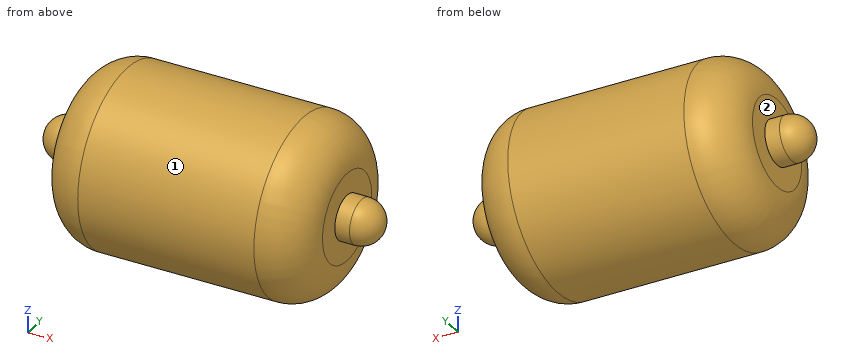
Autodesk Inventor part; units mm, degrees
ref_plane "YZ Plane" through (0, 0, 0) normal (1, 0, 0) x (0, 1, 0)
ref_plane "XZ Plane" through (0, 0, 0) normal (0, 1, 0) x (-1, 0, 0)
ref_plane "XY Plane" through (0, 0, 0) normal (0, 0, 1) x (1, 0, 0)
sketch "Sketch1" plane through (0, 0, 0) normal (0, 0, 1) x (1, 0, 0)
  line L0 (-9, -6) -> (9, -6)
  line L1 (9, -6) -> (9, 6)
  line L2 (9, 6) -> (-9, 6)
  line L3 (-9, 6) -> (-9, 0)
  line L4 (-9, -6) -> (9, 6) construction
  line L5 (9, -6) -> (-9, 6) construction
  line L6 (-9, 0) -> (9, 0)
  point P0 (0, 0)
  dimension "d0" = 18
  dimension "d1" = 12
revolve "Revolution1" add sketch "Sketch1" angle 360 about axis through (-9, 0, 0) along (1, 0, 0)
sketch "Sketch2" plane through (9, 0, 0) normal (1, 0, 0) x (0, 0, -1)
  circle A0 centre (0, 0) radius 1.5
  dimension "d3" = 3
extrude "Extrusion1" add sketch "Sketch2" along normal blind 2.5
fillet "Fillet1" radius 1.5 1 edges at (11.5, 0, 1.5)
mirror "Mirror1" about plane through (0, 0, 0) normal (1, 0, 0) of "Extrusion1"
fillet "Fillet2" radius 1.5 1 edges at (-11.5, 0, 1.5)
fillet "Fillet3" radius 3 2 edges at (-9, -6, 0) (9, -6, 0)
properties part number "roller"
Could you check a few things on this model? Use its own coordinates, in mm. Face numbers are marked on the shaded views. Coordinates: 2 decimals unless noted, no trailing zeros. Order: outer loops, then holes, each group sorted by start corner. A loop starts at its lowest first (then second) coordinate and runs counter-clockwise, first axis right, second up. Notation, with made-up numbers: (-2, -34.75) -> (23, -34.75) arc R23 cw to (23, 4.25) -> close; hole circle Ø11 at (0, -34.5). An arc over 180 degrees is marked (long way). One line per question, with ' | ' between items.
Q1. Thinking about a two-plate mould opening in Y: for the marked faces 1 and 2, which applies, pulls with the +Y half, pulls with the -Y half, needs draft (parallel to the pull), parting line crosses it, or undercut?
Return value:
face 1: parting line crosses it | face 2: needs draft
Q2. If I drill on L1, parallel to X at y = -1, z = 2.25; L2, parallel to Z at x = -1, y = 0.5; L3, parallel to X at y = 3, z = -2.5, over which ranges is the centre line in solid material (lowest first)?
Return value:
L1: -9 to 9 | L2: -5.98 to 5.98 | L3: -8.86 to 8.86
Q3. Imagine slicing it at A-A on x = -1.25. Please give me the cut outline in (y, z), and give its area (3 significant figures).
Return value:
outline: circle Ø12 at (0, 0) | area: 113 mm²
Q4. I'm going to push flat-ended pins straight in: P1, Ø6, axis at x = 2, y = 4.5, coming from the +Z side; P2, Ø1.5, axis at x = 7.5, z = 3, coming from the +Y side; P3, Ø1, axis at y = -3, z = -2.5, coming from the -X side. Where does each tip first touch, or does it pass through?
Return value:
P1: z = 5.81 | P2: y = 5.29 | P3: x = -8.97
Q5. Imagine slicing it at B-B on x = -9.5. Please give me the cut outline in (y, z), and give its area (3 significant figures).
Return value:
outline: circle Ø3 at (0, 0) | area: 7.07 mm²
